The model under review builds one solid part; all positions refer to its coordinate system, in mm. Round coordinates to 2 decimals unless told otherwise and drop trailing zeros. Order: outer loops, then holes, each group sorted by start corner. A loop starts at its lowest first (then second) coordinate and runs counter-clockwise, first axis right, second up. Notation, with made-up numbers: M -21.5,37 L -10.5,37 A24 ccw -10.5,72 Z; hole C 8,5 d4. An arc over 180 degrees is marked long. Answer as a JSON object with one key per item and string values. Group by question number.
1. Clearance check with flat-ended pins moving along their axes: P1, Ø0.7, axis at y = -2, z = 0, coming from the +X side; P2, Ø0.7, axis at x = 0, y = -0.5, coming from the +Z side; P3, Ø1, axis at x = 3.5, z = 0.5, coming from the +Y side. State where each tip first meets the part, or that it passes through.
2. Add section A-A on y = 4.75. State the section outline as (x, z) points.
3. To check wall thickness, follow probe 1 along X at (y, z) = (2.25, -0.55); probe 2 along Z at (x, y) = (8.25, 0.5); probe 3 along Y at (x, z) = (-0.5, -0.45). State the ranges of each line that lie inside material, in increasing order. Write a range as [from, to].
```python
from build123d import *

# Parameters (mm, degrees)
EXTRUDE_2_DEPTH                    = 2.54
EXTRUDE_2_2_DEPTH                  = 2.54
EXTRUDE_2_3_DEPTH                  = 2.54
EXTRUDE_2_4_DEPTH                  = 2.54
EXTRUDE_2_5_DEPTH                  = 2.54
EXTRUDE_2_6_DEPTH                  = 2.54
EXTRUDE_START                      = 0.8
SKETCH_3_W                         = 0.22
SKETCH_3_H                         = 1.34
EXTRUDE_3_DEPTH                    = 1.3
SKETCH_4_W                         = 1.74
SKETCH_4_H                         = 0.54
CUT_EXTRUDE_1_DEPTH                = 16.28610153
EXTRUDE_START_2                    = -3
SKETCH_5_W                         = 0.64
SKETCH_5_H                         = 0.64
EXTRUDE_4_DEPTH                    = 11.54
CHAMFER_1_SIZE                     = 0.2
CHAMFER_2_SIZE                     = 0.2
PATTERN_LINEAR_1_COUNT             = 6
PATTERN_LINEAR_1_PITCH             = 2.54
CHAMFER_1_OF_PATTERN_LINEAR_1_SIZE = 0.2
CHAMFER_2_OF_PATTERN_LINEAR_1_SIZE = 0.2


with BuildPart() as part:
    # Sketch 2 → Extrude 2 (new body)
    with BuildSketch(Plane(origin=(0, 0, 0), x_dir=(1, 0, 0), z_dir=(0, 1, 0))):
        Polygon((-1.05, 0.87), (-0.65, 1.27), (0.65, 1.27), (1.05, 0.87), (1.05, -0.87), (0.65, -1.27), (-0.65, -1.27), (-1.05, -0.87), align=None)
    extrude(amount=EXTRUDE_2_DEPTH)



with BuildPart() as body_2:
    # Sketch 2 → Extrude 2 2 (new body)
    with BuildSketch(Plane(origin=(0, 0, 0), x_dir=(1, 0, 0), z_dir=(0, 1, 0))):
        Polygon((1.89, -1.27), (3.19, -1.27), (3.59, -0.87), (3.59, 0.87), (3.19, 1.27), (1.89, 1.27), (1.49, 0.87), (1.49, -0.87), align=None)
    extrude(amount=EXTRUDE_2_2_DEPTH)


with BuildPart() as body_3:
    # Sketch 2 → Extrude 2 3 (new body)
    with BuildSketch(Plane(origin=(0, 0, 0), x_dir=(1, 0, 0), z_dir=(0, 1, 0))):
        Polygon((4.43, -1.27), (5.73, -1.27), (6.13, -0.87), (6.13, 0.87), (5.73, 1.27), (4.43, 1.27), (4.03, 0.87), (4.03, -0.87), align=None)
    extrude(amount=EXTRUDE_2_3_DEPTH)


with BuildPart() as body_4:
    # Sketch 2 → Extrude 2 4 (new body)
    with BuildSketch(Plane(origin=(0, 0, 0), x_dir=(1, 0, 0), z_dir=(0, 1, 0))):
        Polygon((6.97, -1.27), (8.27, -1.27), (8.67, -0.87), (8.67, 0.87), (8.27, 1.27), (6.97, 1.27), (6.57, 0.87), (6.57, -0.87), align=None)
    extrude(amount=EXTRUDE_2_4_DEPTH)


with BuildPart() as body_5:
    # Sketch 2 → Extrude 2 5 (new body)
    with BuildSketch(Plane(origin=(0, 0, 0), x_dir=(1, 0, 0), z_dir=(0, 1, 0))):
        Polygon((9.51, -1.27), (10.81, -1.27), (11.21, -0.87), (11.21, 0.87), (10.81, 1.27), (9.51, 1.27), (9.11, 0.87), (9.11, -0.87), align=None)
    extrude(amount=EXTRUDE_2_5_DEPTH)


with BuildPart() as body_6:
    # Sketch 2 → Extrude 2 6 (new body)
    with BuildSketch(Plane(origin=(0, 0, 0), x_dir=(1, 0, 0), z_dir=(0, 1, 0))):
        Polygon((12.05, -1.27), (13.35, -1.27), (13.75, -0.87), (13.75, 0.87), (13.35, 1.27), (12.05, 1.27), (11.65, 0.87), (11.65, -0.87), align=None)
    extrude(amount=EXTRUDE_2_6_DEPTH)


with BuildPart() as part_1:
    add(part.part)

    add(body_2.part)  # Extrude 3 merges body 2

    add(body_3.part)  # Extrude 3 merges body 3

    add(body_4.part)  # Extrude 3 merges body 4

    add(body_5.part)  # Extrude 3 merges body 5

    add(body_6.part)  # Extrude 3 merges body 6
    # Sketch 3 → Extrude 3 (add)
    with BuildSketch(Plane(origin=(0, 0, 0), x_dir=(1, 0, 0), z_dir=(0, 1, 0)).offset(EXTRUDE_START)):
        with Locations((-1.16, 0)):
            Rectangle(SKETCH_3_W, SKETCH_3_H)
        with Locations((1.16, 0)):
            Rectangle(SKETCH_3_W, SKETCH_3_H)
        with Locations((1.38, 0)):
            Rectangle(SKETCH_3_W, SKETCH_3_H)
        with Locations((3.7, 0)):
            Rectangle(SKETCH_3_W, SKETCH_3_H)
        with Locations((3.92, 0)):
            Rectangle(SKETCH_3_W, SKETCH_3_H)
        with Locations((6.24, 0)):
            Rectangle(SKETCH_3_W, SKETCH_3_H)
        with Locations((6.46, 0)):
            Rectangle(SKETCH_3_W, SKETCH_3_H)
        with Locations((8.78, 0)):
            Rectangle(SKETCH_3_W, SKETCH_3_H)
        with Locations((11.32, 0)):
            Rectangle(SKETCH_3_W, SKETCH_3_H)
        with Locations((11.54, 0)):
            Rectangle(SKETCH_3_W, SKETCH_3_H)
        with Locations((9, 0)):
            Rectangle(SKETCH_3_W, SKETCH_3_H)
        with Locations((13.86, 0)):
            Rectangle(SKETCH_3_W, SKETCH_3_H)
    extrude(amount=EXTRUDE_3_DEPTH)

    # Sketch 4 → Cut-Extrude 1 (cut, through all)
    with BuildSketch(Plane.ZY.offset(1.05)):
        with Locations((0, 0.27)):
            Rectangle(SKETCH_4_W, SKETCH_4_H)
    extrude(amount=-CUT_EXTRUDE_1_DEPTH, mode=Mode.SUBTRACT)

    # Sketch 5 → Extrude 4 (add)
    with BuildSketch(Plane(origin=(0, 0, 0), x_dir=(1, 0, 0), z_dir=(0, 1, 0)).offset(EXTRUDE_START_2)):
        Rectangle(SKETCH_5_W, SKETCH_5_H)
    extrude_4 = extrude(amount=EXTRUDE_4_DEPTH)

    # Chamfer 1
    chamfer_1_edges = [part_1.edges().sort_by_distance(p)[0] for p in [
        (0.32, 8.54, 0),
        (0, 8.54, -0.32),
        (-0.32, 8.54, 0),
        (0, 8.54, 0.32),
    ]]
    chamfer(chamfer_1_edges, length=CHAMFER_1_SIZE)

    # Chamfer 2
    chamfer_2_edges = [part_1.edges().sort_by_distance(p)[0] for p in [
        (0.32, -3, 0),
        (0, -3, 0.32),
        (-0.32, -3, 0),
        (0, -3, -0.32),
    ]]
    chamfer(chamfer_2_edges, length=CHAMFER_2_SIZE)

    # Pattern Linear 1: Extrude 4 ×6
    with Locations(*[(i * PATTERN_LINEAR_1_PITCH, 0, 0) for i in range(1, PATTERN_LINEAR_1_COUNT)]):
        add(extrude_4)

    # Chamfer 1 of Pattern Linear 1
    chamfer_1_of_pattern_linear_1_edges = [part_1.edges().sort_by_distance(p)[0] for p in [
        (2.86, 8.54, 0),
        (2.54, 8.54, -0.32),
        (2.22, 8.54, 0),
        (2.54, 8.54, 0.32),
        (5.4, 8.54, 0),
        (5.08, 8.54, -0.32),
        (4.76, 8.54, 0),
        (5.08, 8.54, 0.32),
        (7.94, 8.54, 0),
        (7.62, 8.54, -0.32),
        (7.3, 8.54, 0),
        (7.62, 8.54, 0.32),
        (10.48, 8.54, 0),
        (10.16, 8.54, -0.32),
        (9.84, 8.54, 0),
        (10.16, 8.54, 0.32),
        (13.02, 8.54, 0),
        (12.7, 8.54, -0.32),
        (12.38, 8.54, 0),
        (12.7, 8.54, 0.32),
    ]]
    chamfer(chamfer_1_of_pattern_linear_1_edges, length=CHAMFER_1_OF_PATTERN_LINEAR_1_SIZE)

    # Chamfer 2 of Pattern Linear 1
    chamfer_2_of_pattern_linear_1_edges = [part_1.edges().sort_by_distance(p)[0] for p in [
        (2.86, -3, 0),
        (2.54, -3, 0.32),
        (2.22, -3, 0),
        (2.54, -3, -0.32),
        (5.4, -3, 0),
        (5.08, -3, 0.32),
        (4.76, -3, 0),
        (5.08, -3, -0.32),
        (7.94, -3, 0),
        (7.62, -3, 0.32),
        (7.3, -3, 0),
        (7.62, -3, -0.32),
        (10.48, -3, 0),
        (10.16, -3, 0.32),
        (9.84, -3, 0),
        (10.16, -3, -0.32),
        (13.02, -3, 0),
        (12.7, -3, 0.32),
        (12.38, -3, 0),
        (12.7, -3, -0.32),
    ]]
    chamfer(chamfer_2_of_pattern_linear_1_edges, length=CHAMFER_2_OF_PATTERN_LINEAR_1_SIZE)


solid = part_1.part
```
Recorded:
{
 "1": {"P1": "stops at x = 13.02", "P2": "stops at z = 0.32", "P3": "stops at y = 2.54"},
 "2": {"outline": "M -0.32,-0.32 L 0.32,-0.32 L 0.32,0.32 L -0.32,0.32 Z; M 2.22,-0.32 L 2.86,-0.32 L 2.86,0.32 L 2.22,0.32 Z; M 4.76,-0.32 L 5.4,-0.32 L 5.4,0.32 L 4.76,0.32 Z; M 7.3,-0.32 L 7.94,-0.32 L 7.94,0.32 L 7.3,0.32 Z; M 9.84,-0.32 L 10.48,-0.32 L 10.48,0.32 L 9.84,0.32 Z; M 12.38,-0.32 L 13.02,-0.32 L 13.02,0.32 L 12.38,0.32 Z"},
 "3": {"probe 1": "x = [-1.05, 1.05], [1.49, 3.59], [4.03, 6.13], [6.57, 8.67], [9.11, 11.21], [11.65, 13.75]", "probe 2": "z = [-1.27, -0.87], [0.87, 1.27]", "probe 3": "y = [0.54, 2.54]"}
}
